```python
from build123d import *

# Parameters (mm, degrees)
F0_W      = 96
F0_H      = 78
F1_DEPTH  = 18
F2_W      = 72
F2_H      = 39
F3_DEPTH  = 58
F4_W      = 72
F4_H      = 8
F5_DEPTH  = 12
F6_W      = 96
F6_H      = 20
F7_DEPTH  = 5
F10_DEPTH = 39.001
F12_DEPTH = 3
F13_DEPTH = 18.001
F15_DEPTH = 84.001
F16_W     = 72
F16_H     = 17
F17_DEPTH = 3


with BuildPart() as f1:
    # F0 (on Top) → F1 (new body)
    with BuildSketch(Plane.XY):
        with Locations((48, 39)):
            Rectangle(F0_W, F0_H)
    extrude(amount=F1_DEPTH)

    # F2 (on face) → F3 (join)
    with BuildSketch(Plane.XY.offset(18)):
        with Locations((48, 58.5)):
            Rectangle(F2_W, F2_H)
    extrude(amount=F3_DEPTH)

    # F4 (on face) → F5 (cut)
    with BuildSketch(Plane.XY.offset(76)):
        with Locations((48, 51)):
            Rectangle(F4_W, F4_H)
    extrude(amount=-F5_DEPTH, mode=Mode.SUBTRACT)

    # F6 (on face) → F7 (cut)
    with BuildSketch(Plane(origin=(0, 0, 0), x_dir=(1, 0, 0), z_dir=(0, 0, -1))):
        with Locations((48, -20)):
            Rectangle(F6_W, F6_H)
    extrude(amount=-F7_DEPTH, mode=Mode.SUBTRACT)

    # F9 (on face) + F8 (on face) → F10 (cut, through all)
    with BuildSketch(Plane.XZ.offset(-39)):
        Polygon((84, 76), (60, 76), (84, 52), align=None)
    with BuildSketch(Plane(origin=(0, 78, 0), x_dir=(-1, 0, 0), z_dir=(0, 1, 0))):
        Polygon((-84, 18), (-96, 18), (-96, 0), (0, 0), (0, 18), (-12, 18), (-12, 76), (-84, 76), align=None)
    extrude(amount=-F10_DEPTH, dir=(0, -1, 0), mode=Mode.SUBTRACT)

    # F11 (on face) → F12 (join)
    with BuildSketch(Plane.XY.offset(18)):
        with BuildLine():
            ThreePointArc((25, 32.231967628), (12, 19.231967628), (25, 6.231967628))
            Line((25, 6.231967628), (71, 6.231967628))
            ThreePointArc((71, 6.231967628), (84, 19.231967628), (71, 32.231967628))
            Line((71, 32.231967628), (25, 32.231967628))
        make_face()
        with BuildLine():
            Line((71, 13.231967628), (25, 13.231967628))
            ThreePointArc((25, 13.231967628), (19, 19.231967628), (25, 25.231967628))
            Line((25, 25.231967628), (71, 25.231967628))
            ThreePointArc((71, 25.231967628), (77, 19.231967628), (71, 13.231967628))
        make_face(mode=Mode.SUBTRACT)
    extrude(amount=F12_DEPTH)

    # F13 (cut, through all): a face of the model
    f13_faces = [f1.faces().sort_by_distance(p)[0] for p in [
        (48, 19.231967628, 18),
    ]]
    extrude(f13_faces, amount=-F13_DEPTH, mode=Mode.SUBTRACT)

    # F14 (on face) → F15 (cut, through all)
    with BuildSketch(Plane(origin=(12, 0, 0), x_dir=(0, -1, 0), z_dir=(-1, 0, 0))):
        Polygon((-64, 76), (-78, 76), (-78, 40), align=None)
    extrude(amount=-F15_DEPTH, mode=Mode.SUBTRACT)

    # F16 (on face) → F17 (cut)
    with BuildSketch(Plane.XZ.offset(-39)):
        with Locations((48, 26.5)):
            Rectangle(F16_W, F16_H)
    extrude(amount=-F17_DEPTH, mode=Mode.SUBTRACT)


solid = f1.part
```
Could you check a few things on this model? Use its own coordinates, in mm. A direction names the side the tool comes from. Round coordinates to 2 decimals unless told otherwise and drop trailing zeros. Loops run counter-clockwise (first coordinate to the right, second up) from the corner with the lowest first, then second, coordinate; pieces in that order, holes last. Notation, with made-up numbers: M 0.5,88 L 6.5,88 A17 cw 6.5,97 Z; hole C -8,-37.75 d2. An arc over 180 degrees is marked long. Put each result on its own line as item: value.
Q1. On a 3-axis mill with a long thin cutter (end or side, diameter ignored), from which of +Z, -Z, +X, -X, +Y, -Y can I reach the whole of each face in a straight line? I mean faces 1 (the face through (42, 51, 64)), 2 (the face through (47, 28, 21)), 3 (the face through (84, 58, 35)), 4 (the face through (47, 10, 2)), 5 (the face through (48, 13.232, 13)). Say none if no direction works.
Check result:
face 1: +Z, +X, -X
face 2: +Z, +X, -X, -Y
face 3: +Z, +X, +Y, -Y
face 4: -Z, +X, -X
face 5: +Z, -Z
Q2. Imagine slicing it at C-C (y = 18). Write out the boundary of the cut face in (x, z), then the cut area to 3 significant figures.
Check result:
outline: M 0,5 L 19.13,5 L 19.13,21 L 12.06,21 L 12.06,18 L 0,18 Z; M 76.87,5 L 96,5 L 96,18 L 83.94,18 L 83.94,21 L 76.87,21 Z
area: 540 mm2
Q3. Imagine slicing it at B-B (x = 50.5). Write out the boundary of the cut face in (y, z), then the cut area to 3 significant figures.
Check result:
outline: M 0,0 L 10,0 L 10,5 L 13.23,5 L 13.23,21 L 6.23,21 L 6.23,18 L 0,18 Z; M 25.23,5 L 30,5 L 30,0 L 78,0 L 78,40 L 64,76 L 55,76 L 55,64 L 47,64 L 47,76 L 39,76 L 39,35 L 42,35 L 42,18 L 32.23,18 L 32.23,21 L 25.23,21 Z
area: 3,050 mm2
Q4. Thinking about a two-plate mould opening in Y: for faces 6 (the face through (47, 39, 55)), 7 (the face through (96, 38, 9)), 8 (the face through (48, 25.232, 13)), which applies, released by +Y, released by -Y, zero draft, split by the parting line, or undercut?
Check result:
face 6: released by -Y
face 7: zero draft
face 8: undercut
Q5. Imagine slicing it at A-A (z = 8). Write out the boundary of the cut face in (x, y), then the cut area to 3 significant figures.
Check result:
outline: M 0,0 L 96,0 L 96,78 L 0,78 Z; hole M 25,13.23 L 71,13.23 A6 ccw 71,25.23 L 25,25.23 A6 ccw Z
area: 6,820 mm2
Q6. I need wall thicknesses on probe 1 along Y at (x, z) = (33.5, 6.5); probe 2 along Z at (x, y) = (15, 9); probe 3 along X at (y, z) = (69, 21). Which ranges of each line are inside material? Lowest first, please.
Check result:
probe 1: 0 to 13.23, 25.23 to 78
probe 2: 0 to 18
probe 3: 12 to 84
Q7. Imagine slicing it at D-D (z = 66.5). Write out the boundary of the cut face in (x, y).
Check result:
outline: M 12,39 L 69.5,39 L 69.5,47 L 12,47 Z; M 12,55 L 69.5,55 L 69.5,67.69 L 12,67.69 Z
Q8. For pin 1 (16 mm diameter, centred on x = 41.5, y = 17, fed in from -Z); pin 2 (6 mm diameter, centred on y = 41, z = 54.5, fed in from +X); pin 3 (2.5 mm diameter, centred on x = 27, y = 50, fed in from +Z); pin 4 (1 mm diameter, centred on y = 57, z = 48, fed in from -X), each with a flat end and sliding along its axis, tell me the tip position at first contact or that it passes through.
Check result:
pin 1: z = 0
pin 2: x = 84
pin 3: z = 64
pin 4: x = 12
